```python
from build123d import *

# Parameters (mm, degrees)
SKETCH1_W               = 219
SKETCH1_H               = 250
BOSS_EXTRUDE1_DEPTH     = 3
EXTRUDE_THIN1_DEPTH     = 180
CUT_EXTRUDE2_DEPTH      = 256.764051422
CUT_EXTRUDE2_DEPTH_BACK = 256.764051422
SKETCH4_W               = 65.933085688
SKETCH4_H               = 20
SKETCH7_W               = 201
SKETCH7_H               = 9
BOSS_EXTRUDE3_DEPTH     = 40
FILLET7_R               = 5
SKETCH8_W               = 201
SKETCH8_H               = 209
CUT_EXTRUDE3_DEPTH      = 20


with BuildPart() as part:
    # Sketch1 → Boss-Extrude1 (new body)
    with BuildSketch(Plane(origin=(0, 0, 0), x_dir=(1, 0, 0), z_dir=(0, 1, 0))):
        Rectangle(SKETCH1_W, SKETCH1_H)
    extrude(amount=BOSS_EXTRUDE1_DEPTH)

    # Sketch2 → Extrude-Thin1 (add)
    with BuildSketch(Plane(origin=(0, 0, 0), x_dir=(1, 0, 0), z_dir=(0, 1, 0))):
        Polygon((-109.5, -145), (-109.5, -125), (-109.5, 125), (109.5, 125), (109.5, -125), (109.5, -145), (100.5, -145), (100.5, -125), (100.5, 116), (-100.5, 116), (-100.5, -125), (-100.5, -145), align=None)
    extrude(amount=EXTRUDE_THIN1_DEPTH)

    # Sketch4 → Cut-Extrude2 (cut, two sides: drawn at the far end of the back side and taken through both)
    with BuildSketch(Plane(origin=(0, 0, 0), x_dir=(0, 0, -1), z_dir=(1, 0, 0)).offset(-CUT_EXTRUDE2_DEPTH_BACK)):
        with Locations((-134.966542844, 10)):
            Rectangle(SKETCH4_W, SKETCH4_H)
    extrude(amount=CUT_EXTRUDE2_DEPTH + CUT_EXTRUDE2_DEPTH_BACK, mode=Mode.SUBTRACT)

    # Sketch7 → Boss-Extrude3 (add)
    with BuildSketch(Plane(origin=(0, 0, 0), x_dir=(1, 0, 0), z_dir=(0, 1, 0))):
        with Locations((0, -97.5)):
            Rectangle(SKETCH7_W, SKETCH7_H)
    extrude(amount=BOSS_EXTRUDE3_DEPTH)

    # Fillet7
    fillet7_edges = [part.edges().sort_by_distance(p)[0] for p in [
        (-105, 20, 145),
        (105, 20, 145),
    ]]
    fillet(fillet7_edges, radius=FILLET7_R)

    # Sketch8 → Cut-Extrude3 (cut)
    with BuildSketch(Plane(origin=(0, 0, 0), x_dir=(1, 0, 0), z_dir=(0, 1, 0))):
        with Locations((0, 11.5)):
            Rectangle(SKETCH8_W, SKETCH8_H)
    extrude(amount=CUT_EXTRUDE3_DEPTH, mode=Mode.SUBTRACT)


solid = part.part
```
Geometry check sheet. Reference: the model listing, model coordinates, mm. A direction names the side the tool comes from. Give positions to 0.01 mm unless a question says otherwise; leave off trailing zeros. Loops run counter-clockwise (first coordinate to the right, second up) from the corner with the lowest first, then second, coordinate; pieces in that order, holes last. Notation, with made-up numbers: M 23.5,-28.5 L 67.5,-28.5 A20 ccw 67.5,-5.5 Z; hole C 48,-16 d10. An arc over 180 degrees is marked long. Write item = value, one per line. Start each with the question number.
1. Draft check along X on faces 6 (the face through (-106, 0, -12)), 7 (the face through (-109.5, 89, 12)), 8 (the face through (1, 89, -116)). Enter one of: +X half, -X half, draft (parallel to the pull), parting line (faces both ways), or undercut.
2. Section check B-B, the plane z = -83. Enter the section's corners in (x, y).
3. Section check D-D, the plane y = 146.5. Enter the section's corners in (x, z), plus the area to 3 significant figures.
4. Section check C-C, the plane y = 13.5. Enter the section's corners in (x, z).
5. Thickness scan on probe 1 along X at (y, z) = (121, 114); probe 2 along Z at (x, y) = (99.5, 20); probe 3 along Z at (x, y) = (48, 86.5). Record the ranges inside material, lowest first.
6. Tool access check on faces 1 (the face through (109.5, 89, 12)), 2 (the face through (-105, 20, 121)), 3 (the face through (-1, 20, 93)), 4 (the face through (-1, 40, 97)), 5 (the face through (105, 101, 145)). Record the directions out of +Z, -Z, +X, -X, +Y, -Y that give a thin tool (end or side, any length) a straight path to the whole face; none if there is none.
7. Section check A-A, the plane x = -60.5. Enter the section's corners in (y, z).
8. Go/stop test with flat-tipped pins: P1, Ø20, axis at x = -23, y = 10, coming from the +Z side; P2, Ø10, axis at x = -103, z = 126.5, coming from the -Y side; P3, Ø7, axis at x = -4, z = 97, coming from the +Y side. Record where each tip stops, or that it passes through.
Values follow:
q1.face_6 = draft
q1.face_7 = -X half
q1.face_8 = undercut
q2.outline = M -109.5,0 L -100.5,0 L -100.5,180 L -109.5,180 Z; M 100.5,0 L 109.5,0 L 109.5,180 L 100.5,180 Z
q3.outline = M -109.5,-125 L 109.5,-125 L 109.5,145 L 100.5,145 L 100.5,-116 L -100.5,-116 L -100.5,145 L -109.5,145 Z
q3.area = 6,670 mm^2
q4.outline = M -109.5,-125 L 109.5,-125 L 109.5,102 L -109.5,102 Z; hole M -100.5,-116 L 100.5,-116 L 100.5,93 L -100.5,93 Z
q5.probe_1 = -109.5 to -100.5, 100.5 to 109.5
q5.probe_2 = -125 to -116, 93 to 102
q5.probe_3 = -125 to -116
q6.face_1 = +Z, -Z, +X, +Y, -Y
q6.face_2 = +Z, +X, -X, -Y
q6.face_3 = +Y, -Y
q6.face_4 = +Z, +Y
q6.face_5 = +Z, +X, -X, +Y, -Y
q7.outline = M 0,-125 L 180,-125 L 180,-116 L 0,-116 Z; M 0,93 L 40,93 L 40,102 L 0,102 Z
q8.P1 = 102
q8.P2 = 20
q8.P3 = 40
